Could you check a few things on this model? Use its own coordinates, in mm. A direction names the side the tool comes from. Round coordinates to 2 decimals unless told otherwise and drop trailing zeros. Write each loop counter-clockwise with the first axis right and the second up, starting at its lowest first coordinate (ties: lowest second). Pieces come first, ordered by that corner, then holes. Notation, with made-up numbers: (47.25, 69) -> (54.25, 69) arc R12 cw to (54.25, 80) -> close; hole circle Ø4 at (-34.75, -38). An arc over 180 degrees is marked (long way). One line per question, with ' | ' between items. Start each with the question number.
1. Thinking about a two-plate mould opening in Y: for faces 4 (the flat face through (-14, 5, 2)), 5 (the flat face through (-16, 0, 1)), 6 (the flat face through (-95, 13, 2)), 7 (the flat face through (-47.103, -2, 1)), which applies, released by +Y, released by -Y, zero draft, split by the parting line, or undercut?
2. Imagine slicing it at D-D, the plane y = 15.25. List the corners of the cut face in (x, z) for me.
3. If I drill on line 1 along X through (y, z) = (-1.25, 2.25); line 2 along Y through (x, z) = (-65, 1.5); line 3 along Y through (x, z) = (-24, 1.8), over which ranges is the centre line in solid material (lowest first)? Write a range as [from, to].
4. Imagine slicing it at B-B, the plane x = 3. List the corners of the cut face in (y, z) for me.
5. For faces 1 (the flat face through (17, 10, 2)), 2 (the flat face through (-83, -3, 1)), 3 (the flat face through (16, 13, 2)), which set-ups out of +Z, -Z, +X, -X, +Y, -Y let a thin tool reach every point of the face, with its end or its side?
6. Imagine slicing it at C-C, the plane z = 2.05. State how many separate pieces and enclosed holes the cut face has, and give its area (4 significant figures).
7. For pin 1 Ø1 at (x, z) = (-48.5, 1.5) entering from -Y; pin 2 Ø0.9 at (y, z) = (-1.5, 1.5) entering from +X; pin 3 Ø1 at (y, z) = (-2.5, 0.5) entering from -X, each with a flat end and sliding along its axis, tell me the tip position at first contact or that it passes through.
8. Imagine slicing it at A-A, the plane y = 7.5. List the corners of the cut face in (x, z) for me.
from build123d import *

# Parameters (mm, degrees)
BOSS_EXTRUDE1_DEPTH = 3
SKETCH3_W           = 15
SKETCH3_H           = 13
BOSS_EXTRUDE2_DEPTH = 3
SKETCH2_W           = 6
SKETCH2_H           = 5
SKETCH2_W_2         = 5
CUT_EXTRUDE1_DEPTH  = 3
CHAMFER1_SIZE       = 2
SKETCH4_W           = 15
SKETCH4_H           = 3
BOSS_EXTRUDE3_DEPTH = 3


with BuildPart() as part:
    # Sketch1 → Boss-Extrude1 (new body)
    with BuildSketch(Plane.XY):
        Polygon((0, 0), (-78, 0), (-78, -5), (-83, -5), (-83, 0), (-88, 0), (-88, 13), (-78, 18), (0, 18), (10, 13), (10, 0), (5, 0), (5, -5), (0, -5), align=None)
    extrude(amount=BOSS_EXTRUDE1_DEPTH)

    # Sketch3 → Boss-Extrude2 (add)
    with BuildSketch(Plane.XY.offset(3)):
        with Locations((17.5, 6.5)):
            Rectangle(SKETCH3_W, SKETCH3_H)
        with Locations((-95.5, 6.5)):
            Rectangle(SKETCH3_W, SKETCH3_H)
    extrude(amount=-BOSS_EXTRUDE2_DEPTH)

    # Sketch2 → Cut-Extrude1 (cut)
    with BuildSketch(Plane.XY.offset(3)):
        with Locations((-64.5, 7.5)):
            Rectangle(SKETCH2_W, SKETCH2_H)
        with Locations((-13.5, 7.5)):
            Rectangle(SKETCH2_W, SKETCH2_H)
        with Locations((2.5, 7.5)):
            Rectangle(SKETCH2_W_2, SKETCH2_H)
        with Locations((-80.5, 7.5)):
            Rectangle(SKETCH2_W_2, SKETCH2_H)
        with Locations((17.37, 7.5)):
            Rectangle(SKETCH2_W, SKETCH2_H)
        with Locations((-96.83, 7.5)):
            Rectangle(SKETCH2_W, SKETCH2_H)
    extrude(amount=-CUT_EXTRUDE1_DEPTH, mode=Mode.SUBTRACT)

    # Chamfer1
    chamfer1_edges = [part.edges().sort_by_distance(p)[0] for p in [
        (25, 13, 1.5),
        (-103, 13, 1.5),
    ]]
    chamfer(chamfer1_edges, length=CHAMFER1_SIZE)

    # Sketch4 → Boss-Extrude3 (add)
    with BuildSketch(Plane(origin=(0, 0, 0), x_dir=(-1, 0, 0), z_dir=(0, 0, -1))):
        with Locations((39.602582465, -1.5)):
            Rectangle(SKETCH4_W, SKETCH4_H)
    extrude(amount=-BOSS_EXTRUDE3_DEPTH)


solid = part.part
Geometry results:
1) face 4: undercut | face 5: released by -Y | face 6: released by +Y | face 7: zero draft
2) outline: (-83.5, 0) -> (5.5, 0) -> (5.5, 3) -> (-83.5, 3) -> close
3) line 1: x = [-83, -78], [-47.1, -32.1], [0, 5] | line 2: y = [0, 5], [10, 18] | line 3: y = [0, 18]
4) outline: (-5, 0) -> (5, 0) -> (5, 3) -> (-5, 3) -> close; (10, 0) -> (16.5, 0) -> (16.5, 3) -> (10, 3) -> close
5) face 1: +Z, -Z | face 2: +Z, -Z, -X, -Y | face 3: +Z, -Z, +X, +Y
6) separate pieces: 1 | enclosed holes: 6 | area: 2,025 mm2
7) pin 1: stops at y = 0 | pin 2: stops at x = 5 | pin 3: stops at x = -83
8) outline: (-103, 0) -> (-99.83, 0) -> (-99.83, 3) -> (-103, 3) -> close; (-93.83, 0) -> (-83, 0) -> (-83, 3) -> (-93.83, 3) -> close; (-78, 0) -> (-67.5, 0) -> (-67.5, 3) -> (-78, 3) -> close; (-61.5, 0) -> (-16.5, 0) -> (-16.5, 3) -> (-61.5, 3) -> close; (-10.5, 0) -> (0, 0) -> (0, 3) -> (-10.5, 3) -> close; (5, 0) -> (14.37, 0) -> (14.37, 3) -> (5, 3) -> close; (20.37, 0) -> (25, 0) -> (25, 3) -> (20.37, 3) -> close
